from build123d import *

# Parameters (mm, degrees)
F0_R     = 2.5
F1_DEPTH = 2.5


with BuildPart() as f1:
    # F0 (on Front) → F1 (new body, symmetric)
    with BuildSketch(Plane.XZ):
        with BuildLine():
            ThreePointArc((39.691309, -5), (39.9265, -2.504915), (40.005, 0))
            ThreePointArc((40.005, 0), (39.9265, 2.504915), (39.691309, 5))
            ThreePointArc((39.691309, 5), (28.287807, 28.287807), (5, 39.691309))
            ThreePointArc((5, 39.691309), (0, 40.005), (-5, 39.691309))
            ThreePointArc((-5, 39.691309), (-28.287807, 28.287807), (-39.691309, 5))
            ThreePointArc((-39.691309, 5), (-40.005, 0), (-39.691309, -5))
            ThreePointArc((-39.691309, -5), (-28.287807, -28.287807), (-5, -39.691309))
            ThreePointArc((-5, -39.691309), (0, -40.005), (5, -39.691309))
            ThreePointArc((5, -39.691309), (28.287807, -28.287807), (39.691309, -5))
        make_face()
        with BuildLine():
            ThreePointArc((-5, -30.594117), (-21.92031, -21.92031), (-30.594117, -5))
            Line((-30.594117, -5), (-5.59017, -5))
            ThreePointArc((-5.59017, -5), (-5.303301, -5.303301), (-5, -5.59017))
            Line((-5, -5.59017), (-5, -30.594117))
        make_face(mode=Mode.SUBTRACT)
        with BuildLine():
            ThreePointArc((5, -5.59017), (5.303301, -5.303301), (5.59017, -5))
            Line((5.59017, -5), (30.594117, -5))
            ThreePointArc((30.594117, -5), (21.92031, -21.92031), (5, -30.594117))
            Line((5, -30.594117), (5, -5.59017))
        make_face(mode=Mode.SUBTRACT)
        with BuildLine():
            Line((-5, 30.594117), (-5, 5.59017))
            ThreePointArc((-5, 5.59017), (-5.303301, 5.303301), (-5.59017, 5))
            Line((-5.59017, 5), (-30.594117, 5))
            ThreePointArc((-30.594117, 5), (-21.92031, 21.92031), (-5, 30.594117))
        make_face(mode=Mode.SUBTRACT)
        Circle(F0_R, mode=Mode.SUBTRACT)
        with BuildLine():
            Line((30.594117, 5), (5.59017, 5))
            ThreePointArc((5.59017, 5), (5.303301, 5.303301), (5, 5.59017))
            Line((5, 5.59017), (5, 30.594117))
            ThreePointArc((5, 30.594117), (21.92031, 21.92031), (30.594117, 5))
        make_face(mode=Mode.SUBTRACT)
    extrude(amount=F1_DEPTH, both=True)


solid = f1.part
Can you work these out from the model? Positions are in its coordinate system, mm. A direction names the side the tool comes from. Round coordinates to 2 decimals unless told otherwise and drop trailing zeros. Write each loop counter-clockwise with the first axis right and the second up, starting at its lowest first coordinate (ties: lowest second). Pieces come first, ordered by that corner, then holes. Notation, with made-up numbers: M 43,46 L 73,46 A10 ccw 73,53 Z; hole C 70,-23 d11. An arc over 180 degrees is marked long. Use CSV: the item, a comma, the result in double quotes.
(1) Imagine slicing it at B-B (z = 20.5). Write out the boundary of the cut face in (x, y).
Check values:
outline,"M -34.35,-2.5 L -23.25,-2.5 L -23.25,2.5 L -34.35,2.5 Z; M -5,-2.5 L 5,-2.5 L 5,2.5 L -5,2.5 Z; M 23.25,-2.5 L 34.35,-2.5 L 34.35,2.5 L 23.25,2.5 Z"
(2) I'm going to push flat-ended pins straight in: pin 1 (2.5 mm diameter, centred on x = -20, y = -1, fed in from +Z); pin 2 (1.5 mm diameter, centred on y = -2, z = 31, fed in from +X); pin 3 (2 mm diameter, centred on y = -0.5, z = 3, fed in from +X) (3 decimals). Where does each tip first touch, or does it pass through?
Check values:
pin 1,"z = 35.34"
pin 2,"x = 26.18"
pin 3,"x = 39.955"
(3) Imagine slicing it at A-A (x = 0). Write out the boundary of the cut face in (y, z) (3 decimals).
Check values:
outline,"M -2.5,-40.005 L 2.5,-40.005 L 2.5,-2.5 L -2.5,-2.5 Z; M -2.5,2.5 L 2.5,2.5 L 2.5,40.005 L -2.5,40.005 Z"
(4) On a 3-axis mill with a long thin cutter (end or side, diameter ignored), from which of +Z, -Z, +X, -X, +Y, -Y can I reach the whole of each face in a straight line? I mean faces 1 (the flat face through (-5, 0, -18)), 2 (the cylindrical face through (-28.548, -0.035, -28.025)). Say none if no direction works.
Check values:
face 1,"+Y, -Y"
face 2,"-Z, -X, +Y, -Y"
(5) I need wall thicknesses on line 1 along Z through (x, y) = (6.5, -2.15); line 2 along Z through (x, y) = (0, -0.25) (3 decimals); line 3 along X through (y, z) = (0.1, -5.5). Which ranges of each line are inside material? Lowest first, please.
Check values:
line 1,"-39.47 to -30.31, -5 to 5, 30.31 to 39.47"
line 2,"-40.005 to -2.5, 2.5 to 40.005"
line 3,"-39.63 to -30.51, -5.1 to 5.1, 30.51 to 39.63"
(6) Imagine slicing it at D-D (x = 27). Write out the boundary of the cut face in (y, z).
Check values:
outline,"M -2.5,-29.52 L 2.5,-29.52 L 2.5,-15.23 L -2.5,-15.23 Z; M -2.5,-5 L 2.5,-5 L 2.5,5 L -2.5,5 Z; M -2.5,15.23 L 2.5,15.23 L 2.5,29.52 L -2.5,29.52 Z"
(7) We'd pull the mould along X, two halves only. Please class faces 3 (the flat face through (18, 0, 5)), 4 (the flat face through (-1, 2.5, -8)), 5 (the cylindrical face through (28.025, -0.035, -28.548)), 6 (the cylindrical face through (-40.005, -0.035, 0.07)): +X half, -X half, draft (parallel to the pull), parting line (faces both ways), or undercut.
Check values:
face 3,"undercut"
face 4,"draft"
face 5,"+X half"
face 6,"-X half"
(8) Imagine slicing it at C-C (y = 1). Write out the boundary of the cut face in (x, z) (3 decimals).
Check values:
outline,"M -39.691,-5 A40.005 ccw -5,-39.691 A40.005 ccw 5,-39.691 A40.005 ccw 39.691,-5 A40.005 ccw 40.005,0 A40.005 ccw 39.691,5 A40.005 ccw 5,39.691 A40.005 ccw -5,39.691 A40.005 ccw -39.691,5 A40.005 ccw Z; hole M -30.594,-5 A31 ccw -5,-30.594 L -5,-5.59 A7.5 cw -5.59,-5 Z; hole M -30.594,5 L -5.59,5 A7.5 cw -5,5.59 L -5,30.594 A31 ccw Z; hole C 0,0 d5; hole M 5,-30.594 A31 ccw 30.594,-5 L 5.59,-5 A7.5 cw 5,-5.59 Z; hole M 5,5.59 A7.5 cw 5.59,5 L 30.594,5 A31 ccw 5,30.594 Z"
